```python
from build123d import *

# Parameters (mm, degrees)
F0_R     = 4.3815
F0_R_2   = 38.1
F1_DEPTH = 0.762


with BuildPart() as f1:
    # F0 (on Top) → F1 (new body)
    with BuildSketch(Plane.XY):
        with BuildLine():
            Line((-30.618591, -44.45), (30.618591, -44.45))
            ThreePointArc((30.618591, -44.45), (0, 53.975), (-30.618591, -44.45))
        make_face()
        with Locations((-38.93477, -22.479)):
            Circle(F0_R, mode=Mode.SUBTRACT)
        with Locations((38.93477, -22.479)):
            Circle(F0_R, mode=Mode.SUBTRACT)
        Circle(F0_R_2, mode=Mode.SUBTRACT)
        with Locations((0, 44.958)):
            Circle(F0_R, mode=Mode.SUBTRACT)
    extrude(amount=F1_DEPTH)


solid = f1.part
```
Model file for the job. Use its own axes, mm. Give positions to 0.01 mm unless a question says otherwise; leave off trailing zeros. Loops run counter-clockwise (first coordinate to the right, second up) from the corner with the lowest first, then second, coordinate; pieces in that order, holes last. Notation, with made-up numbers: (52.25, -2) -> (107.25, -2) arc R16 ccw to (107.25, 5) -> close; hole circle Ø5 at (70, 78.25). An arc over 180 degrees is marked (long way). Write each question's results on one line, items separated by ' | '.
(1) Cut at C-C on x = 0. Give the number of separate pieces and of enclosed holes in the cut face, and give its area (3 significant figures).
Geometry results:
separate pieces: 3 | enclosed holes: 0 | area: 10.3 mm²
(2) Cut at B-B on x = -23. List the corners of the cut face in (y, z).
Geometry results:
outline: (-44.45, 0) -> (-30.37, 0) -> (-30.37, 0.76) -> (-44.45, 0.76) -> close; (30.37, 0) -> (48.83, 0) -> (48.83, 0.76) -> (30.37, 0.76) -> close
(3) Pull direction X, two halves, no side cores. Call faces 1 (the cylindrical face through (1.92, 53.94, 0.38)), 2 (the cylindrical face through (-36.913, -26.366, 0.376)), 3 (the flat face through (-0.8, 38.3, 0.762)): released by +X, released by -X, zero draft, split by the parting line, or undercut.
Geometry results:
face 1: split by the parting line | face 2: undercut | face 3: zero draft
(4) Probe line 1 along X through (y, z) = (1, 0.35); line 2 along X through (y, z) = (-2.5, 0.25); line 3 along Y through (x, z) = (-26.5, 0.3). List the from-to ranges inside material, lowest first.
Geometry results:
line 1: x = -53.97 to -38.09, 38.09 to 53.97 | line 2: x = -53.92 to -38.02, 38.02 to 53.92 | line 3: y = -44.45 to -27.37, 27.37 to 47.02
(5) Cut at A-A on y = 0. List the corners of the cut face in (x, z) (3 decimals).
Geometry results:
outline: (-53.975, 0) -> (-38.1, 0) -> (-38.1, 0.762) -> (-53.975, 0.762) -> close; (38.1, 0) -> (53.975, 0) -> (53.975, 0.762) -> (38.1, 0.762) -> close
